```python
from build123d import *

# Parameters (mm, degrees)
BASE_FLANGE1_DEPTH  = 2.588
SKETCH2_W           = 2.588
SKETCH2_H           = 72
BOSS_EXTRUDE1_DEPTH = 2.588
SKETCH3_W           = 2.588
SKETCH3_H           = 220
BOSS_EXTRUDE2_DEPTH = 3.264
SKETCH4_W           = 2.588
SKETCH4_H           = 72
BOSS_EXTRUDE3_DEPTH = 2.5888
FILLET1_SIZE        = 5


# Sheet-metal steps are written as plain solids
with BuildPart() as part:
    # Base-Flange1: sheet metal written as solids
    # Sketch1 → Base-Flange1 (new body)
    with BuildSketch(Plane(origin=(0, 0, 0), x_dir=(0, 0, -1), z_dir=(1, 0, 0))):
        Polygon((0, 172), (46.072551481, 198.6), (67, 198.6), (67, 156.6), (378.084, 156.6), (378.084, 198.6), (429.151448519, 198.6), (475.224, 172), (475.224, 0), (0, 0), align=None)
    extrude(amount=-BASE_FLANGE1_DEPTH)

    # Sketch2 → Boss-Extrude1 (add)
    with BuildSketch(Plane(origin=(0, 0, -475.224), x_dir=(-1, 0, 0), z_dir=(0, 0, -1))):
        with Locations((1.294, 126)):
            Rectangle(SKETCH2_W, SKETCH2_H)
        with Locations((1.294, 46)):
            Rectangle(SKETCH2_W, SKETCH2_H)
    extrude(amount=BOSS_EXTRUDE1_DEPTH)

    # Sketch3 → Boss-Extrude2 (add)
    with BuildSketch(Plane.XZ):
        with Locations((-1.294, -122)):
            Rectangle(SKETCH3_W, SKETCH3_H)
        with Locations((-1.294, -353.224)):
            Rectangle(SKETCH3_W, SKETCH3_H)
    extrude(amount=BOSS_EXTRUDE2_DEPTH)

    # Sketch4 → Boss-Extrude3 (add)
    with BuildSketch(Plane.XY):
        with Locations((-1.294, 126)):
            Rectangle(SKETCH4_W, SKETCH4_H)
        with Locations((-1.294, 46)):
            Rectangle(SKETCH4_W, SKETCH4_H)
    extrude(amount=BOSS_EXTRUDE3_DEPTH)

    # Fillet1
    # a fillet whose section is not a circle: 5 mm, written as the material it takes off along each edge
    with BuildSketch(Plane(origin=(12.5, 198.6, -378.084), x_dir=(0, -1, 0), z_dir=(-1, 0, 0)), Plane(origin=(12.5, 198.6, -67), x_dir=(0, 0, 1), z_dir=(-1, 0, 0))) as fillet1_piece_1:
        with BuildLine():
            add(Edge.make_bspline([(FILLET1_SIZE, 0), (4.159009742, 0), (3.318019485, 0), (1.464466094, -0.358459599), (0.358459599, -1.464466094), (0, -3.318019485), (0, -4.159009742), (0, -FILLET1_SIZE)], knots=[0, 0, 0, 0, 0, 0, 0.5, 0.5, 1, 1, 1, 1, 1, 1], degree=5))
            Line((0, -FILLET1_SIZE), (0, 0))
            Line((0, 0), (FILLET1_SIZE, 0))
        make_face()
    extrude(amount=27.588, mode=Mode.SUBTRACT)
    with BuildSketch(Plane(origin=(3.349364905, 198.6, -429.151448519), x_dir=(0, 0, 1), z_dir=(-1, 0, 0)), Plane(origin=(3.349364905, 198.6, -46.072551481), x_dir=(0, -0.49999999999999534, 0.8660254037844413), z_dir=(-1, 0, 0))) as fillet1_piece_2:
        with BuildLine():
            add(Edge.make_bspline([(1.339745962, 0), (1.091155955, 0), (0.842565948, 0), (0.288878575, -0.029943211), (-0.235204579, -0.170370869), (-0.729683516, -0.421282974), (-0.944968777, -0.545577978), (-1.160254038, -0.669872981)], knots=[0, 0, 0, 0, 0, 0, 0.5, 0.5, 1, 1, 1, 1, 1, 1], degree=5))
            Line((-1.160254038, -0.669872981), (0, 0))
            Line((0, 0), (1.339745962, 0))
        make_face()
    extrude(amount=9.286729811, mode=Mode.SUBTRACT)


solid = part.part
```
Part model, mm, in its own coordinate system. Give positions to 0.01 mm unless a question says otherwise; leave off trailing zeros. Write each loop counter-clockwise with the first axis right and the second up, starting at its lowest first coordinate (ties: lowest second). Pieces come first, ordered by that corner, then holes. Notation, with made-up numbers: (-33.5, 12) -> (-23.5, 12) arc R14 cw to (-23.5, 30) -> close; hole circle Ø2 at (39, 45). An arc over 180 degrees is marked (long way). Put each result on its own line as item: value. Start each with the question number.
Item 1: Wall check: L1, parallel to Z at x = -0.2, y = 161.5; L2, parallel to Z at x = -0.3, y = 164.5; L3, parallel to Y at x = -2.1, z = -289.5. Give the ranges that are in metal, low to high. Write a range as [from, to].
Item 2: Cut at A-A (z = -302). List the corners of the cut face in (x, y).
Item 3: Pin check, flat tips, straight feed: pin 1 Ø1.3 at (x, y) = (-1, -2) entering from +Z; pin 2 Ø1.3 at (x, y) = (-2, 165) entering from -Z; pin 3 Ø0.8 at (x, y) = (-1.5, -1) entering from -Z. Stop position of each tip, or through.
Item 4: Cut at B-B (z = -33). List the corners of the cut face in (x, y), then the cut area to 3 significant figures.
Answer list:
1. L1: z = [-477.81, -378.08], [-67, 2.59]
1. L2: z = [-475.22, -378.08], [-67, 0]
1. L3: y = [-3.26, 156.6]
2. outline: (-2.59, -3.26) -> (0, -3.26) -> (0, 156.6) -> (-2.59, 156.6) -> close
3. pin 1: stops at z = -12
3. pin 2: stops at z = -475.22
3. pin 3: stops at z = -463.22
4. outline: (-2.59, -3.26) -> (0, -3.26) -> (0, 191.05) -> (-2.59, 191.05) -> close
4. area: 503 mm2
